Build history of the part. All positions in model axes, mm. A direction names the side the tool comes from. Give positions to 0.01 mm unless a question says otherwise; leave off trailing zeros. Order: outer loops, then holes, each group sorted by start corner. A loop starts at its lowest first (then second) coordinate and runs counter-clockwise, first axis right, second up. Notation, with made-up numbers: (-20, 12) - (-12, 12) arc R26 ccw to (-12, 27) - close; hole circle Ø3 at (35.5, 17). An arc over 180 degrees is marked (long way). One line per item, written item: value.
```python
from build123d import *

# Parameters (mm, degrees)
F0_W            = 30
F0_H            = 15
F0_H_2          = 50
F0_H_3          = 25.4
F1_DEPTH        = 15
F2_DEPTH        = 38.1
F5_W            = 38.1
F5_H            = 15
F6_ANGLE        = 60
F7_DEPTH        = 61
F8_DEPTH        = 15
F9_W            = 30
F9_H            = 15
F10_DEPTH       = 25.4
F12_DEPTH       = 26.924
F14_D           = 5.08
F14_CBORE_D     = 10.16
F14_CBORE_DEPTH = 6.35
F15_D           = 5.08
F15_CBORE_D     = 10.16
F15_CBORE_DEPTH = 6.35
F17_DEPTH       = 60.96
F18_DEPTH       = 45.212
F19_SIZE        = 5.08


# Not quite as in the source:
# - a feature of the source that left no trace in its solid (it failed there, or was rolled back) is left out


with BuildPart() as f1:
    # F0 (on Front) → F1 (new body)
    with BuildSketch(Plane.XZ):
        with Locations((-21.4830274055, 50.8597951472)):
            Rectangle(F0_W, F0_H)
        with Locations((-21.4830274055, 18.3597951472)):
            Rectangle(F0_W, F0_H_2)
        with Locations((-21.4830274055, -19.3402048528)):
            Rectangle(F0_W, F0_H_3)
    extrude(amount=F1_DEPTH)

    # F0 (on Front) → F2 (join)
    with BuildSketch(Plane.XZ):
        with Locations((-21.4830274055, 50.8597951472)):
            Rectangle(F0_W, F0_H)
    extrude(amount=-F2_DEPTH)

    # F5 (on face) → F6 (revolve)
    with BuildSketch(Plane.YZ.offset(-6.4830274055)):
        with Locations((19.05, 50.8597951472)):
            Rectangle(F5_W, F5_H)
    revolve(axis=Axis((-6.4830274055, 0, 50.8597951472), (0, 0, -1)), revolution_arc=F6_ANGLE)

    # F0 (on Front) → F7 (join)
    with BuildSketch(Plane.XZ):
        with Locations((-21.4830274055, -19.3402048528)):
            Rectangle(F0_W, F0_H_3)
    extrude(amount=F7_DEPTH)

    # F8 (add): a face of the model
    f8_faces = [f1.faces().sort_by_distance(p)[0] for p in [
        (-21.4830274055, -61, -19.3402048528),
    ]]
    extrude(f8_faces, amount=F8_DEPTH)

    # F9 (on face) → F10 (join)
    with BuildSketch(Plane.XY.offset(-6.6402048528)):
        with Locations((-21.4830274055, -68.5)):
            Rectangle(F9_W, F9_H)
    extrude(amount=F10_DEPTH)

    # F11 (on face) → F12 (cut)
    with BuildSketch(Plane.XY.offset(58.3597951472)):
        with BuildLine():
            Line((-6.4830274055, 38.1), (-6.4830274055, 0))
            Line((-6.4830274055, 0), (26.5125404787, 19.05))
            ThreePointArc((26.5125404787, 19.05), (12.5669725945, 32.9955678842), (-6.4830274055, 38.1))
        make_face()
    extrude(amount=-F12_DEPTH, mode=Mode.SUBTRACT)

    # F14 (through all)
    with Locations(Plane.XY.offset(58.3597951472)):
        with Locations((-21.4830274055, 24.5092792876)):
            CounterBoreHole(F14_D / 2, F14_CBORE_D / 2, F14_CBORE_DEPTH)

    # F15 (through all)
    with Locations(Plane.XY.offset(58.3597951472)):
        with Locations((-21.4830274055, 10.9185585752)):
            CounterBoreHole(F15_D / 2, F15_CBORE_D / 2, F15_CBORE_DEPTH)

    # F16 (on face) → F17 (cut)
    with BuildSketch(Plane.YZ.offset(-6.4830274055)):
        Polygon((0, -18.8376810402), (-69.65, -18.8376810402), (-76, -18.8376810402), (-76, -32.0402048528), (0, -32.0402048528), align=None)
        Polygon((13.4356496856, -18.8376810402), (0, -18.8376810402), (0, -32.0402048528), (-76, -32.0402048528), (-76, -18.8376810402), (-82.0414423943, -18.8376810402), (-82.0414423943, -58.5641600192), (13.4356496856, -58.5641600192), align=None)
    extrude(amount=-F17_DEPTH, mode=Mode.SUBTRACT)

    # F16 (on face) → F18 (cut)
    with BuildSketch(Plane.YZ.offset(-6.4830274055)):
        Polygon((13.4356496856, -18.8376810402), (0, -18.8376810402), (0, -32.0402048528), (-76, -32.0402048528), (-76, -18.8376810402), (-82.0414423943, -18.8376810402), (-82.0414423943, -58.5641600192), (13.4356496856, -58.5641600192), align=None)
        Polygon((0, -18.8376810402), (-69.65, -18.8376810402), (-76, -18.8376810402), (-76, -32.0402048528), (0, -32.0402048528), align=None)
    extrude(amount=-F18_DEPTH, mode=Mode.SUBTRACT)

    # F19
    f19_edges = [f1.edges().sort_by_distance(p)[0] for p in [
        (-6.483027, -38, -6.640205),
        (-36.483027, -38, -6.640205),
        (-36.483027, -68.5, 18.759795),
        (-21.483027, -76, 18.759795),
        (-6.483027, -68.5, 18.759795),
        (-21.483027, -61, 18.759795),
        (-36.483027, -76, -0.038943),
        (-6.483027, -76, -0.038943),
        (-21.483027, -76, -18.837681),
        (-6.483027, -38, -18.837681),
        (-36.483027, -38, -18.837681),
        (-21.483027, 0, -18.837681),
        (-21.483027, -15, 58.359795),
        (-6.483027, -15, 25.859795),
        (-21.483027, -15, -6.640205),
        (-36.483027, -15, 25.859795),
        (-6.483027, -61, 6.059795),
        (-36.483027, -61, 6.059795),
        (-21.483027, -61, -6.640205),
        (-6.483027, 11.55, 58.359795),
        (-36.483027, 11.55, 58.359795),
        (-21.483027, 38.1, 58.359795),
        (-6.483027, 0, 12.261057),
        (-36.483027, 0, 12.261057),
        (-6.483027, 38.1, 50.859795),
        (-36.483027, 38.1, 50.859795),
    ]]
    chamfer(f19_edges, length=F19_SIZE)


solid = f1.part
```
(1) Slice it at A-A, the plane z = 24.5. Give the cut face in (x, y), and give its area (3 significant figures).
Completed:
outline: (-36.48, -9.92) - (-31.4, -15) - (-11.56, -15) - (-6.48, -9.92) - (-6.48, -5.08) - (-11.56, 0) - (-31.4, 0) - (-36.48, -5.08) - close
area: 398 mm²
(2) Slice it at C-C, the plane y = -42. Give the cut face in (x, z).
Completed:
outline: (-36.48, -13.76) - (-31.4, -18.84) - (-11.56, -18.84) - (-6.48, -13.76) - (-6.48, -11.72) - (-11.56, -6.64) - (-31.4, -6.64) - (-36.48, -11.72) - close
(3) Pin check, flat tips, straight feed: P1, Ø2, axis at x = -18.5, y = -32.5, coming from the +Z side; P2, Ø6, axis at x = -28, z = 14, coming from the +Y side; P3, Ø4.5, axis at x = -21.48, y = 10.92, coming from the +Z side (3 decimals); P4, Ø8, axis at x = -21.48, y = 10.92, coming from the +Z side. Stop position of each tip, or through.
Completed:
P1: z = -6.64
P2: y = 0
P3: through
P4: z = 52.01
(4) Slice it at B-B, the plane x = -20.5. Count the separate pieces of the cut face and the enclosed holes in it, and give its area (3 significant figures).
Completed:
separate pieces: 3
enclosed holes: 0
area: 2,600 mm²
(5) 3-axis set-ups, long thin cutter, end or side, ignore diameter. For faces 5 (the face through (-22, -61, 6)), 6 (the face through (-8.987, -2.576, 15.201)), 7 (the face through (-10.03, -64.14, 15.29)), 8 (the face through (-20, 27, 52.01)), 9 (the face through (-33.907, 35.596, 48.25)): which of +Z, -Z, +X, -X, +Y, -Y reach the whole face in a straight line?
Completed:
face 5: +Z, +X, -X
face 6: -Z, +X, +Y
face 7: +Z, +X
face 8: +Z
face 9: +Z, -Z, -X, +Y
(6) Drill centre lines: line 1 (Y direction, x = -23, z = 10); line 2 (Z direction, x = -13, y = -69); line 3 (Y direction, x = -15, z = 16). Where is each one in solid material? Low to high.
Completed:
line 1: -76 to -61, -15 to 0
line 2: -18.84 to 18.76
line 3: -73.68 to -63.32, -15 to 0
(7) Pull direction Y, two halves, no side cores. Call faces 1 (the face through (-21.34, -2.5, -16.26)), 2 (the face through (-32.937, -64.14, 15.285)), 3 (the face through (-10.029, -72.526, -15.698)), 4 (the face through (-33.907, -63.504, 5.953)): +Y half, -Y half, draft (parallel to the pull), parting line (faces both ways), or undercut.
Completed:
face 1: +Y half
face 2: undercut
face 3: -Y half
face 4: undercut
(8) Slice it at D-D, the plane x = -34. Give the cut face in (y, z), and give its area (3 significant figures).
Completed:
outline: (-73.4, -13.76) - (-70.92, -16.24) - (-5.08, -16.24) - (-2.6, -13.76) - (-2.6, 43.36) - (35.5, 43.36) - (35.5, 53.28) - (33.02, 55.76) - (-9.92, 55.76) - (-12.4, 53.28) - (-12.4, -1.56) - (-20.08, -9.24) - (-55.92, -9.24) - (-63.6, -1.56) - (-63.6, 13.68) - (-66.08, 16.16) - (-70.92, 16.16) - (-73.4, 13.68) - close
area: 1,900 mm²
